Part model, mm, in its own coordinate system. A direction names the side the tool comes from. Give positions to 0.01 mm unless a question says otherwise; leave off trailing zeros. Write each loop counter-clockwise with the first axis right and the second up, starting at its lowest first coordinate (ties: lowest second). Pieces come first, ordered by that corner, then holes. Notation, with made-up numbers: M 48,58.25 L 55,58.25 A16 ccw 55,68.25 Z; hole C 87.5,46.5 d6. An arc over 180 degrees is marked long. Use a Markdown table: item, result.
```python
from build123d import *

# Parameters (mm, degrees)
F0_R     = 0.585
F1_DEPTH = 9.3
F2_DEPTH = 1
F3_DEPTH = 8.3
F4_R     = 0.45
F5_DEPTH = 9.301


# Not quite as in the source:
# - a feature names something its author has since deleted; it is built from what else it names


with BuildPart() as f1:
    # F0 (on Top) → F1 (new body)
    with BuildSketch(Plane.XY):
        with BuildLine():
            Line((0, 1.21), (-3.2, 1.21))
            ThreePointArc((-3.2, 1.21), (-3.8050588257, 1.0478567734), (-4.2479586591, 0.6048823429))
            Line((-4.2479586591, 0.6048823429), (-5.0479586591, -0.7811176571))
            ThreePointArc((-5.0479586591, -0.7811176571), (-5.21, -1.386), (-5.0479586591, -1.9908823429))
            Line((-5.0479586591, -1.9908823429), (-4.2479586591, -3.3768823429))
            ThreePointArc((-4.2479586591, -3.3768823429), (-3.8050588257, -3.8198567734), (-3.2, -3.982))
            Line((-3.2, -3.982), (0, -3.982))
            ThreePointArc((0, -3.982), (0.8555992052, -3.6275992052), (1.21, -2.772))
            Line((1.21, -2.772), (1.21, 0))
            ThreePointArc((1.21, 0), (0.8555992052, 0.8555992052), (0, 1.21))
        make_face()
        with BuildLine():
            ThreePointArc((-3.8149178909, 0.3549309616), (-3.5550345175, 0.6148581067), (-3.2, 0.71))
            Line((-3.2, 0.71), (0, 0.71))
            ThreePointArc((0, 0.71), (0.5020458146, 0.5020458146), (0.71, 0))
            Line((0.71, 0), (0.71, -2.772))
            ThreePointArc((0.71, -2.772), (0.5020458146, -3.2740458146), (0, -3.482))
            Line((0, -3.482), (-3.2, -3.482))
            ThreePointArc((-3.2, -3.482), (-3.5550345175, -3.3868581067), (-3.8149178909, -3.1269309616))
            Line((-3.8149178909, -3.1269309616), (-4.6149178909, -1.7409309616))
            ThreePointArc((-4.6149178909, -1.7409309616), (-4.71, -1.386), (-4.6149178909, -1.0310690384))
            Line((-4.6149178909, -1.0310690384), (-3.8149178909, 0.3549309616))
        make_face(mode=Mode.SUBTRACT)
        with BuildLine():
            Line((0, 0.71), (-3.2, 0.71))
            ThreePointArc((-3.2, 0.71), (-3.5550345175, 0.6148581067), (-3.8149178909, 0.3549309616))
            Line((-3.8149178909, 0.3549309616), (-4.6149178909, -1.0310690384))
            ThreePointArc((-4.6149178909, -1.0310690384), (-4.71, -1.386), (-4.6149178909, -1.7409309616))
            Line((-4.6149178909, -1.7409309616), (-3.8149178909, -3.1269309616))
            ThreePointArc((-3.8149178909, -3.1269309616), (-3.5550345175, -3.3868581067), (-3.2, -3.482))
            Line((-3.2, -3.482), (0, -3.482))
            ThreePointArc((0, -3.482), (0.5020458146, -3.2740458146), (0.71, -2.772))
            Line((0.71, -2.772), (0.71, 0))
            ThreePointArc((0.71, 0), (0.5020458146, 0.5020458146), (0, 0.71))
        make_face()
        with Locations((-3.2, -2.772)):
            Circle(F0_R, mode=Mode.SUBTRACT)
        with Locations((-4, -1.386)):
            Circle(F0_R, mode=Mode.SUBTRACT)
        with Locations((-2.4, -1.386)):
            Circle(F0_R, mode=Mode.SUBTRACT)
        with Locations((-1.6, -2.772)):
            Circle(F0_R, mode=Mode.SUBTRACT)
        with Locations((0, -2.772)):
            Circle(F0_R, mode=Mode.SUBTRACT)
        with Locations((-0.8, -1.386)):
            Circle(F0_R, mode=Mode.SUBTRACT)
        with Locations((-3.2, 0)):
            Circle(F0_R, mode=Mode.SUBTRACT)
        with Locations((-1.6, 0)):
            Circle(F0_R, mode=Mode.SUBTRACT)
        Circle(F0_R, mode=Mode.SUBTRACT)
        with Locations((-4, -1.386)):
            Circle(F0_R)
        with Locations((-3.2, 0)):
            Circle(F0_R)
        with Locations((-1.6, 0)):
            Circle(F0_R)
        with Locations((-2.4, -1.386)):
            Circle(F0_R)
        with Locations((-3.2, -2.772)):
            Circle(F0_R)
        with Locations((-1.6, -2.772)):
            Circle(F0_R)
        with Locations((-0.8, -1.386)):
            Circle(F0_R)
        Circle(F0_R)
        with Locations((0, -2.772)):
            Circle(F0_R)
    extrude(amount=-F1_DEPTH)

    # F0 (on Top) → F2 (cut)
    with BuildSketch(Plane.XY):
        with BuildLine():
            Line((0, 0.71), (-3.2, 0.71))
            ThreePointArc((-3.2, 0.71), (-3.5550345175, 0.6148581067), (-3.8149178909, 0.3549309616))
            Line((-3.8149178909, 0.3549309616), (-4.6149178909, -1.0310690384))
            ThreePointArc((-4.6149178909, -1.0310690384), (-4.71, -1.386), (-4.6149178909, -1.7409309616))
            Line((-4.6149178909, -1.7409309616), (-3.8149178909, -3.1269309616))
            ThreePointArc((-3.8149178909, -3.1269309616), (-3.5550345175, -3.3868581067), (-3.2, -3.482))
            Line((-3.2, -3.482), (0, -3.482))
            ThreePointArc((0, -3.482), (0.5020458146, -3.2740458146), (0.71, -2.772))
            Line((0.71, -2.772), (0.71, 0))
            ThreePointArc((0.71, 0), (0.5020458146, 0.5020458146), (0, 0.71))
        make_face()
        with Locations((-3.2, -2.772)):
            Circle(F0_R, mode=Mode.SUBTRACT)
        with Locations((-4, -1.386)):
            Circle(F0_R, mode=Mode.SUBTRACT)
        with Locations((-2.4, -1.386)):
            Circle(F0_R, mode=Mode.SUBTRACT)
        with Locations((-1.6, -2.772)):
            Circle(F0_R, mode=Mode.SUBTRACT)
        with Locations((0, -2.772)):
            Circle(F0_R, mode=Mode.SUBTRACT)
        with Locations((-0.8, -1.386)):
            Circle(F0_R, mode=Mode.SUBTRACT)
        with Locations((-3.2, 0)):
            Circle(F0_R, mode=Mode.SUBTRACT)
        with Locations((-1.6, 0)):
            Circle(F0_R, mode=Mode.SUBTRACT)
        Circle(F0_R, mode=Mode.SUBTRACT)
        Circle(F0_R)
        with Locations((-0.8, -1.386)):
            Circle(F0_R)
        with Locations((0, -2.772)):
            Circle(F0_R)
        with Locations((-4, -1.386)):
            Circle(F0_R)
        with Locations((-2.4, -1.386)):
            Circle(F0_R)
        with Locations((-3.2, 0)):
            Circle(F0_R)
        with Locations((-1.6, 0)):
            Circle(F0_R)
        with Locations((-1.6, -2.772)):
            Circle(F0_R)
        with Locations((-3.2, -2.772)):
            Circle(F0_R)
    extrude(amount=-F2_DEPTH, mode=Mode.SUBTRACT)

    # F0 (on Top) → F3 (cut)
    with BuildSketch(Plane.XY):
        with Locations((-0.8, -1.386)):
            Circle(F0_R)
        Circle(F0_R)
        with Locations((0, -2.772)):
            Circle(F0_R)
        with Locations((-1.6, -2.772)):
            Circle(F0_R)
        with Locations((-3.2, -2.772)):
            Circle(F0_R)
        with Locations((-2.4, -1.386)):
            Circle(F0_R)
        with Locations((-1.6, 0)):
            Circle(F0_R)
        with Locations((-3.2, 0)):
            Circle(F0_R)
        with Locations((-4, -1.386)):
            Circle(F0_R)
    extrude(amount=-F3_DEPTH, mode=Mode.SUBTRACT)

    # F4 (on Top) → F5 (cut, through all)
    with BuildSketch(Plane.XY):
        with Locations((-3.2, 0)):
            Circle(F4_R)
        with Locations((-1.6, 0)):
            Circle(F4_R)
        Circle(F4_R)
        with Locations((-0.8, -1.386)):
            Circle(F4_R)
        with Locations((-2.4, -1.386)):
            Circle(F4_R)
        with Locations((-4, -1.386)):
            Circle(F4_R)
        with Locations((-3.2, -2.772)):
            Circle(F4_R)
        with Locations((-1.6, -2.772)):
            Circle(F4_R)
        with Locations((0, -2.772)):
            Circle(F4_R)
    extrude(amount=-F5_DEPTH, mode=Mode.SUBTRACT)


solid = f1.part
```
1. Two-plate mould, pull along Y, no slides. Class faces 3 (the cylindrical face through (-5.21, -1.38, -4.58)), 4 (the flat face through (-4.642, -0.078, -4.585)), 5 (the flat face through (-1.4, -0.9, -1)), 6 (the cylindrical face through (-2.771, 0.135, -8.793)): released by +Y, released by -Y, zero draft, split by the parting line, or undercut.
Findings below:
| item | result |
|---|---|
| face 3 | split by the parting line |
| face 4 | released by +Y |
| face 5 | undercut |
| face 6 | undercut |
2. Drill centre lines: L1, parallel to Y at x = -3.2, z = -9; L2, parallel to Y at x = -3.2, z = -7 (3 decimals); L3, parallel to X at y = -1.35, z = -0.25. Where is each one in solid material? Low to high.
Findings below:
| item | result |
|---|---|
| L1 | -3.98 to -3.22, -2.32 to -0.45, 0.45 to 1.21 |
| L2 | -3.982 to -3.357, -2.187 to -0.585, 0.585 to 1.21 |
| L3 | -5.21 to -4.71, 0.71 to 1.21 |
3. Cut at D-D, the plane z = -0.75. Give the cut face in (x, y).
Findings below:
| item | result |
|---|---|
| outline | M -5.05,-1.99 L -4.25,-3.38 A1.21 ccw -3.2,-3.98 L 0,-3.98 A1.21 ccw 1.21,-2.77 L 1.21,0 A1.21 ccw 0,1.21 L -3.2,1.21 A1.21 ccw -4.25,0.6 L -5.05,-0.78 A1.21 ccw Z; hole M -4.61,-1.74 L -3.81,-3.13 A0.71 ccw -3.2,-3.48 L 0,-3.48 A0.71 ccw 0.71,-2.77 L 0.71,0 A0.71 ccw 0,0.71 L -3.2,0.71 A0.71 ccw -3.81,0.35 L -4.61,-1.03 A0.71 ccw Z |
4. Cut at C-C, the plane y = -2.6. State how many separate pieces and enclosed holes the cut face has, then the cut area to 3 significant figures.
Findings below:
| item | result |
|---|---|
| separate pieces | 4 |
| enclosed holes | 0 |
| area | 23.1 mm2 |
5. Cut at A-A, the plane x = -1.6. Give the cut face in (y, z) (3 decimals).
Findings below:
| item | result |
|---|---|
| outline | M -3.982,-9.3 L -3.222,-9.3 L -3.222,-8.3 L -3.357,-8.3 L -3.357,-1 L -3.482,-1 L -3.482,0 L -3.982,0 Z; M -2.322,-9.3 L -0.45,-9.3 L -0.45,-8.3 L -0.585,-8.3 L -0.585,-1 L -2.187,-1 L -2.187,-8.3 L -2.322,-8.3 Z; M 0.45,-9.3 L 1.21,-9.3 L 1.21,0 L 0.71,0 L 0.71,-1 L 0.585,-1 L 0.585,-8.3 L 0.45,-8.3 Z |
6. Drop flat-ended pins along their axis: P1, Ø0.6, axis at x = -3, y = 0, coming from the +Z side; P2, Ø0.9, axis at x = -1.5, y = -3, coming from the +Z side. Give the stop position or say it passes through.
Findings below:
| item | result |
|---|---|
| P1 | z = -8.3 |
| P2 | z = -1 |
7. Tool access for faces 1 (the cylindrical face through (-4.584, -1.36, -4.599)), 2 (the cylindrical face through (-2.99, -3.17, -8.79)): list every direction of +Z, -Z, +X, -X, +Y, -Y with a clear straight run to the whole face (end or side of a thin tool).
Findings below:
| item | result |
|---|---|
| face 1 | +Z |
| face 2 | +Z, -Z |
8. Cut at B-B, the plane x = -2.4. Give the cut face in (y, z).
Findings below:
| item | result |
|---|---|
| outline | M -3.98,-9.3 L -1.84,-9.3 L -1.84,-8.3 L -1.97,-8.3 L -1.97,-1 L -3.48,-1 L -3.48,0 L -3.98,0 Z; M -0.94,-9.3 L 1.21,-9.3 L 1.21,0 L 0.71,0 L 0.71,-1 L -0.8,-1 L -0.8,-8.3 L -0.94,-8.3 Z |
